The listing builds one solid part. Answer for the finished solid, in the listing's coordinates (mm). Coordinates: 2 decimals unless noted, no trailing zeros. Order: outer loops, then holes, each group sorted by start corner. A loop starts at its lowest first (then second) coordinate and runs counter-clockwise, first axis right, second up. Notation, with made-up numbers: (79.25, 53) - (103.25, 53) arc R32 cw to (103.25, 85) - close; hole circle Ø9 at (-9.5, -28.75). An arc over 180 degrees is marked (long way). Use a Markdown table: item, result. Add a question column.
Item 1: The part is cut by section D-D, the plane x = -9.5. Give the vertices of the cut face in (y, z) (3 decimals), then the cut area to 3 significant figures.
Item 2: The part is cut by section B-B, the plane x = 57. Give the vertices of the cut face in (y, z).
Item 3: Flat-ended cylindrical pins translate along their axes: P1, Ø10, axis at y = 4, z = 39, coming from the +X side; P2, Ø12, axis at y = 12, z = 42.5, coming from the +X side; P3, Ø2, axis at y = 0, z = 14.5, coming from the -X side. Find the tip coordinate at first contact, or state that the pin passes through.
Item 4: The mould has two halves that part along Y. Classify faces 1 (the flat face through (-37, -12, 49.318)), 2 (the cylindrical face through (-78.203, 1.274, 29.794)), 3 (the cylindrical face through (27.997, 0.7, 12.522)): released by +Y, released by -Y, zero draft, split by the parting line, or undercut.
Item 5: The part is cut by section A-A, the plane y = 0. Give the vertices of the cut face in (x, z), then the cut area to 3 significant figures.
Item 6: Find the intervals of material crossed by line 1 along Z through (x, y) = (11.5, -9.5); line 2 along Y through (x, z) = (-39.5, 28); line 3 along X through (y, z) = (-11, 29.5), in increasing order.
Item 7: The part is cut by section C-C, the plane z = 13. State how many separate pieces and enclosed holes the cut face has, then the cut area to 3 significant figures.
from build123d import *

# Parameters (mm, degrees)
F0_R     = 15.9205
F1_DEPTH = 25.4
F2_DEPTH = 49.318


# Not quite as in the source:
# - a feature names something its author has since deleted; it is built from what else it names


with BuildPart() as f1:
    # F0 (on Top) → F1 (new body)
    with BuildSketch(Plane.XY):
        with BuildLine():
            Line((-49.2564179003, -28.975), (43.9025820997, -28.975))
            ThreePointArc((43.9025820997, -28.975), (72.8775820997, 0), (43.9025820997, 28.975))
            Line((43.9025820997, 28.975), (-49.2564179003, 28.975))
            ThreePointArc((-49.2564179003, 28.975), (-28.7679989154, 20.4884189849), (-20.2814179003, 0))
            ThreePointArc((-20.2814179003, 0), (-28.7679989154, -20.4884189849), (-49.2564179003, -28.975))
        make_face()
        with Locations((43.9025820997, 0)):
            Circle(F0_R, mode=Mode.SUBTRACT)
        with BuildLine():
            ThreePointArc((-49.2564179003, 28.975), (-78.2314179003, 0), (-49.2564179003, -28.975))
            ThreePointArc((-49.2564179003, -28.975), (-28.7679989154, -20.4884189849), (-20.2814179003, 0))
            ThreePointArc((-20.2814179003, 0), (-28.7679989154, 20.4884189849), (-49.2564179003, 28.975))
        make_face()
        with Locations((-49.2564179003, 0)):
            Circle(F0_R, mode=Mode.SUBTRACT)
    extrude(amount=F1_DEPTH)

    # F0 (on Top) → F2 (join)
    with BuildSketch(Plane.XY):
        with BuildLine():
            ThreePointArc((-49.2564179003, 28.975), (-78.2314179003, 0), (-49.2564179003, -28.975))
            ThreePointArc((-49.2564179003, -28.975), (-28.7679989154, -20.4884189849), (-20.2814179003, 0))
            ThreePointArc((-20.2814179003, 0), (-28.7679989154, 20.4884189849), (-49.2564179003, 28.975))
        make_face()
        with Locations((-49.2564179003, 0)):
            Circle(F0_R, mode=Mode.SUBTRACT)
    extrude(amount=F2_DEPTH)


solid = f1.part
Solution:
| question | item | result |
|---|---|---|
| 1 | outline | (-28.975, 0) - (28.975, 0) - (28.975, 25.4) - (-28.975, 25.4) - close |
| 1 | area | 1,470 mm2 |
| 2 | outline | (-25.85, 0) - (-9.05, 0) - (-9.05, 25.4) - (-25.85, 25.4) - close; (9.05, 0) - (25.85, 0) - (25.85, 25.4) - (9.05, 25.4) - close |
| 3 | P1 | stops at x = -20.28 |
| 3 | P2 | stops at x = -20.91 |
| 3 | P3 | stops at x = -78.23 |
| 4 | face 1 | zero draft |
| 4 | face 2 | split by the parting line |
| 4 | face 3 | undercut |
| 5 | outline | (-78.23, 0) - (-65.18, 0) - (-65.18, 49.32) - (-78.23, 49.32) - close; (-33.34, 0) - (27.98, 0) - (27.98, 25.4) - (-20.28, 25.4) - (-20.28, 49.32) - (-33.34, 49.32) - close; (59.82, 0) - (72.88, 0) - (72.88, 25.4) - (59.82, 25.4) - close |
| 5 | area | 2,850 mm2 |
| 6 | line 1 | z = 0 to 25.4 |
| 6 | line 2 | y = -27.28 to -12.58, 12.58 to 27.28 |
| 6 | line 3 | x = -76.06 to -60.77, -37.75 to -22.45 |
| 7 | separate pieces | 1 |
| 7 | enclosed holes | 2 |
| 7 | area | 6,440 mm2 |
